from build123d import *

# Parameters (mm, degrees)
F1_DEPTH = 15.24
F2_T     = -2.54
F3_R     = 5.08
F5_D     = 18.47
F5_DEPTH = 14
F5_TIP   = 5.5489478167
F6_W     = 5.08
F6_H     = 90.6730847065
F7_DEPTH = 43.688
F8_W     = 64.9396401966
F8_H     = 5.08
F9_DEPTH = 25.4


with BuildPart() as f1:
    # F0 (on Front) → F1 (new body)
    with BuildSketch(Plane.XZ):
        Polygon((102.5888894677, 61.8790130322), (-94.0111105323, 61.8790130322), (-94.0111105323, -79.4209869678), (-31.6111105323, -79.4209869678), (-31.6111105323, 21.8790130322), (102.5888894677, 21.8790130322), align=None)
    extrude(amount=F1_DEPTH)

    # F2
    f2_openings = [f1.faces().sort_by_distance(p)[0] for p in [
        (100.16779, -15.24, 41.879013),
    ]]
    offset(amount=F2_T, openings=f2_openings, kind=Kind.INTERSECTION)

    # F3
    f3_edges = [f1.edges().sort_by_distance(p)[0] for p in [
        (-94.011111, -7.62, 61.879013),
        (102.588889, -7.62, 61.879013),
        (102.588889, -7.62, 21.879013),
        (-31.611111, -7.62, -79.420987),
        (-94.011111, -7.62, -79.420987),
        (-94.011111, 0, -8.770987),
        (-31.611111, 0, -28.770987),
        (35.488889, 0, 21.879013),
        (4.288889, 0, 61.879013),
        (-62.811111, 0, -79.420987),
        (102.588889, 0, 41.879013),
    ]]
    fillet(f3_edges, radius=F3_R)

    # F5
    with Locations(Plane.YZ.offset(102.5888894677)):
        with Locations((-15.24, 41.8790130322)):
            Hole(F5_D / 2, depth=F5_DEPTH)
            with Locations((0, 0, -(F5_DEPTH + F5_TIP / 2))):  # 118° drill point
                Cone(0, F5_D / 2, F5_TIP, mode=Mode.SUBTRACT)

    # F6 (on face) → F7 (cut)
    with BuildSketch(Plane.YZ.offset(-31.6111105323)):
        with Locations((-12.7, -23.4575293211)):
            Rectangle(F6_W, F6_H)
    extrude(amount=-F7_DEPTH, mode=Mode.SUBTRACT)

    # F8 (on face) → F9 (cut)
    with BuildSketch(Plane(origin=(0, 0, 21.8790130322), x_dir=(1, 0, 0), z_dir=(0, 0, -1))):
        with Locations((-1.681290434, 12.7)):
            Rectangle(F8_W, F8_H)
    extrude(amount=-F9_DEPTH, mode=Mode.SUBTRACT)


solid = f1.part
Can you work these out from the model? Positions are in its coordinate system, mm. A direction names the side the tool comes from. Coordinates: 2 decimals unless noted, no trailing zeros. Write each loop counter-clockwise with the first axis right and the second up, starting at its lowest first coordinate (ties: lowest second). Pieces come first, ordered by that corner, then holes. Notation, with made-up numbers: (44.25, 32) - (100.25, 32) arc R18 ccw to (100.25, 64) - close; hole circle Ø4 at (39, 39.5). An arc over 180 degrees is marked (long way). Return JSON: item names as keys, results as strings. Group by question number.
Item 1: I'm going to push flat-ended pins straight in: pin 1 Ø5 at (x, y) = (39, -7.5) entering from -Z; pin 2 Ø1 at (y, z) = (-2.5, 4.5) entering from +X; pin 3 Ø12 at (x, z) = (59.5, 44.5) entering from -Y. Where does each tip first touch, or does it pass through?
Item 2: Which directions (+Z, -Z, +X, -X, +Y, -Y) give clear straight access to the entire face, cutting with the end or side of a thin tool? Please do faces 1 (the face through (31.348, -1.528, 23.328)), 2 (the face through (-34.151, -6, -27)), 3 (the face through (101.301, -6.007, 42.082)).
Item 3: If we section it at B-B (z = -51.5): Write out the boundary of the cut face in (x, y).
Item 4: Please list where these lines run through material, in increasing order: probe 1 along X at (y, z) = (-9.25, -26); probe 2 along Z at (x, y) = (-20, -7.75); probe 3 along Z at (x, y) = (-76, -9.75).
Item 5: If we section it at A-A (x = 15): Write out the boundary of the cut face in (y, z).
Item 6: If we section it at C-C (y = -8): Write out the boundary of the cut face in (x, z).
Item 7: We'd pull the mould along X, two halves only. Please class faces 4 (the face through (-33.06, -1.53, -22.98)), 5 (the face through (-94.011, -10, -8)), 6 (the face through (-40, -2.54, 7)): pulls with the +X half, pulls with the -X half, needs draft (parallel to the pull), parting line crosses it, or undercut.
Return value:
{
 "1": {"pin 1": "stops at z = 21.88", "pin 2": "stops at x = -32.06", "pin 3": "stops at y = -2.54"},
 "2": {"face 1": "-Z, +X, +Y", "face 2": "-Y", "face 3": "+X, -Y"},
 "3": {"outline": "(-94.01, -15.24) - (-91.47, -15.24) - (-91.47, -2.54) - (-34.15, -2.54) - (-34.15, -10.16) - (-31.61, -10.16) - (-31.61, -5.08) arc R5.08 ccw to (-36.69, 0) - (-88.93, 0) arc R5.08 ccw to (-94.01, -5.08) - close"},
 "4": {"probe 1": "x = -94.01 to -91.47, -34.15 to -31.61", "probe 2": "z = 21.88 to 24.42, 59.34 to 61.88", "probe 3": "z = -79.42 to -76.88, 59.34 to 61.88"},
 "5": {"outline": "(-15.24, 59.34) - (-2.54, 59.34) - (-2.54, 24.42) - (-10.16, 24.42) - (-10.16, 21.88) - (-5.08, 21.88) arc R5.08 ccw to (0, 26.96) - (0, 56.8) arc R5.08 ccw to (-5.08, 61.88) - (-15.24, 61.88) - close"},
 "6": {"outline": "(-94.01, -74.34) arc R5.08 ccw to (-88.93, -79.42) - (-36.69, -79.42) arc R5.08 ccw to (-31.61, -74.34) - (-31.61, 21.88) - (97.51, 21.88) arc R5.08 ccw to (102.59, 26.96) - (102.59, 36.15) - (100.05, 36.15) - (100.05, 24.42) - (-34.15, 24.42) - (-34.15, -76.88) - (-91.47, -76.88) - (-91.47, 59.34) - (100.05, 59.34) - (100.05, 47.61) - (102.59, 47.61) - (102.59, 56.8) arc R5.08 ccw to (97.51, 61.88) - (-88.93, 61.88) arc R5.08 ccw to (-94.01, 56.8) - close"},
 "7": {"face 4": "pulls with the +X half", "face 5": "pulls with the -X half", "face 6": "undercut"}
}
